Geometry: final body of the model. Coordinates: model frame, mm. A direction names the side the tool comes from. Give positions to 0.01 mm unless a question says otherwise; leave off trailing zeros. Write each loop counter-clockwise with the first axis right and the second up, starting at its lowest first coordinate (ties: lowest second). Pieces come first, ordered by that corner, then holes. Notation, with made-up numbers: M 12,45.25 L 49,45.25 A27 ccw 49,74.25 Z; hole C 32,-37 d10. An arc over 180 degrees is marked long. Use a Markdown table: item, result. Add a question column.
(1) Pin query (flat end, axial travel): pin 1 Ø4 at (x, z) = (-83, -6) entering from -Y; pin 2 Ø2 at (x, y) = (-78.5, -16.5) entering from +Z; pin 3 Ø3.5 at (x, y) = (-80.14, -19.26) entering from +Z. Return the tip coordinate at first contact, or that it passes through.
(2) Draft query along Y for faces 1 (the cylindrical face through (-78.75, -19.83, -2.6)), 2 (the cylindrical face through (-78.75, -19.83, 2.58)), 3 (the flat face through (-85.136, -17, 2)), 4 (the cylindrical face through (-76.15, -10.47, -1.95)). Return one class per face: released by +Y, released by -Y, zero draft, split by the parting line, or undercut.
(3) Cut plane D-D (z = 3). Output: boundary loops of the cut face in (x, y), plus the area to 3 significant figures.
(4) Cut plane C-C (x = -80.75). Output: boundary loops of the cut face in (y, z), plus the area to 3 significant figures.
(5) Reachability of faces 5 (the cylindrical face through (-80.066, -17.025, 0.293)), 6 (the flat face through (-83.136, -19, -4)) from +Z, -Z, +X, -X, +Y, -Y: full face, straight path, thin tool, end or side. Return the list, or none.
(6) Cut plane B-B (y = -21). Output: boundary loops of the cut face in (x, z).
(7) Cut plane A-A (z = 0). Output: boundary loops of the cut face in (x, y), plus the area to 3 significant figures.
(8) Material intervals for L1, parallel to X at y = -23.5, z = 4; L2, parallel to Y at x = -81.25, z = 0; L3, parallel to Y at x = -76.75, z = 0, sorted ascending.
```python
from build123d import *

# Parameters (mm, degrees)
SKETCH2_R               = 2.25
CUT_EXTRUDE1_DEPTH      = 32.295394302
CUT_EXTRUDE2_DEPTH      = 91.152948551
CUT_EXTRUDE2_DEPTH_BACK = 91.152948551
SKETCH5_R               = 1.5


with BuildPart() as part:
    # Sketch1 → Revolve2 (revolve)
    with BuildSketch(Plane.XY, mode=Mode.PRIVATE) as revolve2_sk:
        Polygon((-85.136081821, -10.256002982), (-85.136081821, -19.256002982), (-75.136081821, -19.256002982), (-75.136081821, -10.256002982), (-77.136081821, -10.256002982), (-77.136081821, -15.756002982), (-83.136081821, -15.756002982), (-83.136081821, -10.256002982), align=None)
    revolve(revolve2_sk.sketch.rotate(Axis((-85.136081821, -19.256002982, 0), (1, 0, 0)), 90), axis=Axis((-85.136081821, -19.256002982, 0), (1, 0, 0)))

    # Sketch2 → Cut-Extrude1 (cut, through all)
    with BuildSketch(Plane(origin=(-75.136081821, 0, 0), x_dir=(0, 0, -1), z_dir=(1, 0, 0))):
        with Locations((0, -19.256002982)):
            Circle(SKETCH2_R)
    extrude(amount=-CUT_EXTRUDE1_DEPTH, mode=Mode.SUBTRACT)

    # Sketch5 → Cut-Extrude2 (cut, two sides: drawn at the far end of the back side and taken through both)
    with BuildSketch(Plane.XY.offset(-CUT_EXTRUDE2_DEPTH_BACK)):
        with Locations((-80.136081821, -19.256002982)):
            Circle(SKETCH5_R)
    extrude(amount=CUT_EXTRUDE2_DEPTH + CUT_EXTRUDE2_DEPTH_BACK, mode=Mode.SUBTRACT)


solid = part.part
```
Answer list:
| question | item | result |
|---|---|---|
| 1 | pin 1 | y = -27.32 |
| 1 | pin 2 | z = 3.03 |
| 1 | pin 3 | z = 3.5 |
| 2 | face 1 | undercut |
| 2 | face 2 | undercut |
| 2 | face 3 | zero draft |
| 2 | face 4 | split by the parting line |
| 3 | outline | M -85.14,-27.74 L -83.14,-27.74 L -83.14,-21.06 L -77.14,-21.06 L -77.14,-27.74 L -75.14,-27.74 L -75.14,-10.77 L -77.14,-10.77 L -77.14,-17.45 L -83.14,-17.45 L -83.14,-10.77 L -85.14,-10.77 Z; hole C -80.14,-19.26 d3 |
| 3 | area | 82.4 mm² |
| 4 | outline | M -20.62,-3.22 L -20.62,-1.79 A2.25 cw -20.62,1.79 L -20.62,3.22 A3.5 ccw Z; M -17.89,-3.22 A3.5 ccw -17.89,3.22 L -17.89,1.79 A2.25 cw -17.89,-1.79 Z |
| 4 | area | 15.4 mm² |
| 5 | face 5 | +X, -X |
| 5 | face 6 | none |
| 6 | outline | M -85.14,-8.83 L -83.14,-8.83 L -83.14,-3.03 L -77.14,-3.03 L -77.14,-8.83 L -75.14,-8.83 L -75.14,-1.42 L -85.14,-1.42 Z; M -85.14,1.42 L -75.14,1.42 L -75.14,8.83 L -77.14,8.83 L -77.14,3.03 L -83.14,3.03 L -83.14,8.83 L -85.14,8.83 Z |
| 7 | outline | M -85.14,-28.26 L -83.14,-28.26 L -83.14,-22.76 L -77.14,-22.76 L -77.14,-28.26 L -75.14,-28.26 L -75.14,-21.51 L -85.14,-21.51 Z; M -85.14,-17.01 L -75.14,-17.01 L -75.14,-10.26 L -77.14,-10.26 L -77.14,-15.76 L -83.14,-15.76 L -83.14,-10.26 L -85.14,-10.26 Z |
| 7 | area | 69.0 mm² |
| 8 | L1 | -85.14 to -83.14, -77.14 to -75.14 |
| 8 | L2 | -22.76 to -21.51, -17.01 to -15.76 |
| 8 | L3 | -28.26 to -21.51, -17.01 to -10.26 |
